The drawing under review shows one solid part. Ordinate dimensions are in mm from its lowest x, y, z. A direction names the side the tool comes from. Round coordinates to 2 decimals unless told otherwise and drop trailing zeros. Loops run counter-clockwise (first coordinate to the right, second up) from the corner with the lowest first, then second, coordinate; pieces in that order, holes last. Notation, with made-up numbers: M 15.5,16.25 L 57.5,16.25 A28 cw 57.5,47.25 Z; hole C 13.25,-22 d5. An arc over 180 degrees is marked long. Use a Markdown table: item, result.
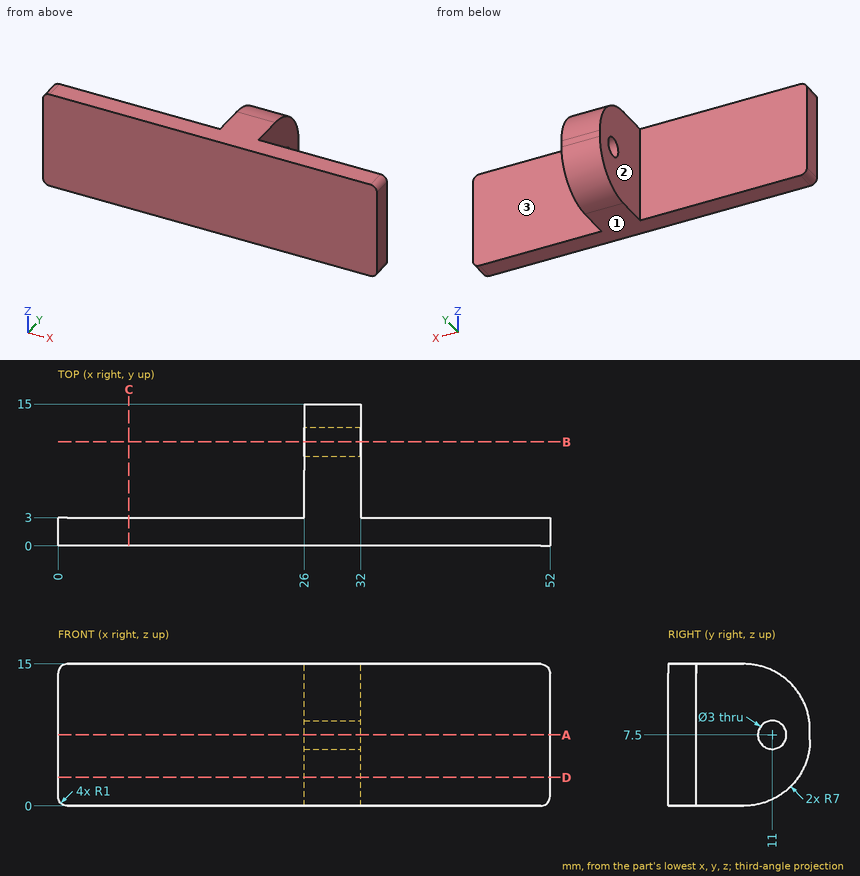
1. Take a section at C-C on x = 7.5. Give the boundary of the cut face in (y, z), and give its area (3 significant figures).
Check values:
| item | result |
|---|---|
| outline | M 0,0 L 3,0 L 3,15 L 0,15 Z |
| area | 45.0 mm² |
2. Take a section at B-B on y = 11. Give the boundary of the cut face in (x, z), and give its area (3 significant figures).
Check values:
| item | result |
|---|---|
| outline | M 26,0.68 L 32,0.68 L 32,6 L 26,6 Z; M 26,9 L 32,9 L 32,14.32 L 26,14.32 Z |
| area | 63.9 mm² |
3. Take a section at A-A on z = 7.5. Give the boundary of the cut face in (x, y), and give its area (3 significant figures).
Check values:
| item | result |
|---|---|
| outline | M 0,0 L 52,0 L 52,3 L 32,3 L 32,9.5 L 26,9.5 L 26,3 L 0,3 Z; M 26,12.5 L 32,12.5 L 32,15 L 26,15 Z |
| area | 210 mm² |
4. Insertion check: pin 1 (6 mm diameter, centred on x = 19, z = 8.5, fed in from +Y); pin 2 (3.5 mm diameter, centred on y = 11, z = 7.5, fed in from +X). Each pin has a flat end and moves straight along its axis. Give the tip position at first contact, or say it passes through.
Check values:
| item | result |
|---|---|
| pin 1 | stops at y = 3 |
| pin 2 | stops at x = 32 |
5. Wall thickness on line 1 along X through (y, z) = (8.5, 6.25); line 2 along Z through (x, y) = (28.5, 11); line 3 along Y through (x, z) = (39.5, 13): over which ranges is each line inside the solid? List them lowest first. Write a range as from..to.
Check values:
| item | result |
|---|---|
| line 1 | x = 26..32 |
| line 2 | z = 0.68..6, 9..14.32 |
| line 3 | y = 0..3 |
6. Take a section at D-D on z = 3. Give the boundary of the cut face in (x, y), and give its area (3 significant figures).
Check values:
| item | result |
|---|---|
| outline | M 0,0 L 52,0 L 52,3 L 32,3 L 32,13.74 L 26,13.74 L 26,3 L 0,3 Z |
| area | 220 mm² |
7. Machinability: for the marked faces 1, 2 and 3, which of the approach directions +Z, -Z, +X, -X, +Y, -Y give a long, thin tool a straight path to every point of the face, cutting with its end or side? Answer none if there is none.
Check values:
| item | result |
|---|---|
| face 1 | -Z, +X, -X, +Y, -Y |
| face 2 | +Z, -Z, -X, +Y |
| face 3 | +Z, -Z, +X, +Y |
